```python
from build123d import *

# Parameters (mm, degrees)
SKETCH2_W                = 12.5
SKETCH2_H                = 12.5
SKETCH2_W_2              = 11.1
SKETCH2_H_2              = 11.1
BOSS_EXTRUDE1_DEPTH      = 105
SKETCH3_R                = 4
CUT_EXTRUDE1_DEPTH       = 105
SKETCH4_W                = 10
SKETCH4_H                = 2
BOSS_EXTRUDE2_DEPTH      = 25
FILLET1_R                = 5
SKETCH5_R                = 2
CUT_EXTRUDE2_DEPTH       = 40
BOSS_EXTRUDE3_START      = -82.5
SKETCH6_R                = 4
BOSS_EXTRUDE3_DEPTH      = 90.5
SKETCH8_W                = 12.5
SKETCH8_H                = 12.5
SKETCH8_W_2              = 11.1
SKETCH8_H_2              = 11.1
BOSS_EXTRUDE4_DEPTH      = 24
BOSS_EXTRUDE5_DEPTH      = 10
BOSS_EXTRUDE5_DEPTH_BACK = 51.049582
SKETCH9_W                = 12.5
SKETCH9_H                = 12.5
SKETCH9_W_2              = 10
SKETCH9_H_2              = 10
SKETCH11_R               = 4
BOSS_EXTRUDE6_DEPTH      = 11
SKETCH12_R               = 4
BOSS_EXTRUDE7_DEPTH      = 11


with BuildPart() as part:
    # Sketch2 → Boss-Extrude1 (new body)
    with BuildSketch(Plane.XY):
        Rectangle(SKETCH2_W, SKETCH2_H)
        Rectangle(SKETCH2_W_2, SKETCH2_H_2, mode=Mode.SUBTRACT)
    extrude(amount=BOSS_EXTRUDE1_DEPTH)

    # Sketch3 → Cut-Extrude1 (cut)
    with BuildSketch(Plane(origin=(0, 6.25, 0), x_dir=(1, 0, 0), z_dir=(0, 1, 0))):
        with Locations(Location((0, -95, 0), (0, 0, 180))):
            Circle(SKETCH3_R)
    extrude(amount=-CUT_EXTRUDE1_DEPTH, mode=Mode.SUBTRACT)

    # Sketch4 → Boss-Extrude2 (add, symmetric)
    with BuildSketch(Plane(origin=(0, 0, 0), x_dir=(0, 0, -1), z_dir=(1, 0, 0))):
        with Locations((-5, 0)):
            Rectangle(SKETCH4_W, SKETCH4_H)
    extrude(amount=BOSS_EXTRUDE2_DEPTH, both=True)

    # Fillet1
    fillet1_edges = [part.edges().sort_by_distance(p)[0] for p in [
        (-25, 0, 10),
        (-25, 0, 0),
        (25, 0, 10),
        (25, 0, 0),
    ]]
    fillet(fillet1_edges, radius=FILLET1_R - 0.0001)  # a hair under: the kernel refuses the full size

    # Sketch5 → Cut-Extrude2 (cut)
    with BuildSketch(Plane(origin=(0, 1, 0), x_dir=(1, 0, 0), z_dir=(0, 1, 0))):
        with Locations(Location((20, -5, 0), (0, 0, 270))):
            Circle(SKETCH5_R)
    cut_extrude2 = extrude(amount=-CUT_EXTRUDE2_DEPTH, mode=Mode.SUBTRACT)

    # Mirror1: Cut-Extrude2 across plane
    add(cut_extrude2.mirror(Plane(origin=(0, 0, 0), x_dir=(0, 0, 1), z_dir=(1, 0, 0))), mode=Mode.SUBTRACT)


with BuildPart() as body_2:
    # Mirror3: mirrored copy
    add(part.part.mirror(Plane(origin=(0, -75, 0), x_dir=(0, 0, 1), z_dir=(0, -1, 0))))



with BuildPart() as part_1:
    add(part.part)

    # Sketch6 → Boss-Extrude3 (add)
    with BuildSketch(Plane(origin=(0, 6.25, 0), x_dir=(1, 0, 0), z_dir=(0, 1, 0)).offset(BOSS_EXTRUDE3_START)):
        with Locations(Location((0, -43, 0), (0, 0, 180))):
            Circle(SKETCH6_R)
    boss_extrude3 = extrude(amount=BOSS_EXTRUDE3_DEPTH)

    # Mirror4: Boss-Extrude3 across plane
    add(boss_extrude3.mirror(Plane(origin=(0, -75, 0), x_dir=(0, 0, 1), z_dir=(0, -1, 0))))

    # Sketch8 → Boss-Extrude4 (add)
    with BuildSketch(Plane(origin=(0, 6.25, 0), x_dir=(1, 0, 0), z_dir=(0, 1, 0))):
        with Locations((0, -60.200417772)):
            Rectangle(SKETCH8_W, SKETCH8_H)
        with Locations((0, -60.200417772)):
            Rectangle(SKETCH8_W_2, SKETCH8_H_2, mode=Mode.SUBTRACT)
    extrude(amount=BOSS_EXTRUDE4_DEPTH)

    # Sketch9 → Boss-Extrude5 (add, two sides: drawn at the far end of the back side and taken through both)
    with BuildSketch(Plane(origin=(0, 0, 53.950417772), x_dir=(-1, 0, 0), z_dir=(0, 0, -1)).offset(-BOSS_EXTRUDE5_DEPTH_BACK)):
        with Locations((0, 36.5)):
            Rectangle(SKETCH9_W, SKETCH9_H)
        with Locations((0, 36.5)):
            Rectangle(SKETCH9_W_2, SKETCH9_H_2, mode=Mode.SUBTRACT)
    extrude(amount=BOSS_EXTRUDE5_DEPTH + BOSS_EXTRUDE5_DEPTH_BACK)

    # Sketch11 → Boss-Extrude6 (add, symmetric)
    with BuildSketch(Plane(origin=(0, 0, 0), x_dir=(1, 0, 0), z_dir=(0, 1, 0))):
        with Locations(Location((0, -95, 0), (0, 0, 180))):
            Circle(SKETCH11_R)
    extrude(amount=BOSS_EXTRUDE6_DEPTH, both=True)


with BuildPart() as body_2_1:
    add(body_2.part)

    add(part_1.part)  # Boss-Extrude7 merges part
    # Sketch12 → Boss-Extrude7 (add, symmetric)
    with BuildSketch(Plane(origin=(0, -150, 0), x_dir=(-1, 0, 0), z_dir=(0, -1, 0))):
        with Locations((0, -95)):
            Circle(SKETCH12_R)
    extrude(amount=BOSS_EXTRUDE7_DEPTH, both=True)


solid = body_2_1.part
```
Geometry: final body of the model. Coordinates: model frame, mm. A direction names the side the tool comes from. Coordinates: 2 decimals unless noted, no trailing zeros. Loops run counter-clockwise (first coordinate to the right, second up) from the corner with the lowest first, then second, coordinate; pieces in that order, holes last. Notation, with made-up numbers: (21.5, 4.25) -> (72.5, 4.25) arc R18 cw to (72.5, 9.25) -> close; hole circle Ø3 at (-28, 34.25). An arc over 180 degrees is marked (long way). Use a Markdown table: item, result. Add a question column.
(1) Section query A-A, the plane z = 51. Return loops of the section in (x, y), plus the area to 3 significant figures.
(2) Section query B-B, the plane x = -11. Return loops of the section in (y, z), plus the area to 3 significant figures.
(3) Line query: line 1 along Y through (x, z) = (-4.5, 46); line 2 along X through (y, z) = (-149.4, 5); line 3 along Y through (x, z) = (5.5, 16). Output: solid intervals per line, ascending.
(4) Section query D-D, the plane x = 0. State how many separate pieces and enclosed holes the cut face has, plus the area to 3 significant figures.
(5) Pin query (flat end, axial travel): pin 1 Ø9 at (x, y) = (1, 19) entering from +Z; pin 2 Ø10 at (x, y) = (0, 21) entering from -Z; pin 3 Ø10 at (x, y) = (0, -75.5) entering from -Z. Return the tip coordinate at first contact, or that it passes through.
(6) Access query for faces 4 (the cylindrical face through (-1.846, -8.592, 91.451)), 5 (the cylindrical face through (-1.846, -158.658, 98.549)), 6 (the flat face through (16, -149, 5)), 7 (the flat face through (-15, -1, 5)), 8 (the flat face through (0, 41.5, 75)). Directions: +Z, -Z, +X, -X, +Y, -Y. A direction counts if a zero-diameter tool reaches every point of the face in a straight line with its end or side. Return the directions, or none.
(7) Mould query, pull axis X, two halves, no side actions, for faces 1 (the cylindrical face through (-22, -150, 5)), 2 (the cylindrical face through (-24, 0, 2)), 3 (the flat face through (0, -11, 95)). Classes: pulls with the +X half, pulls with the -X half, needs draft (parallel to the pull), parting line crosses it, or undercut.
(8) Section query C-C, the plane y = -8.5. Return loops of the section in (x, z), plus the area to 3 significant figures.
Answer:
| question | item | result |
|---|---|---|
| 1 | outline | (-6.25, -156.25) -> (6.25, -156.25) -> (6.25, -143.75) -> (-6.25, -143.75) -> close; (-6.25, -6.25) -> (6.25, -6.25) -> (6.25, 6.25) -> (-6.25, 6.25) -> close; (-6.25, 30.25) -> (6.25, 30.25) -> (6.25, 42.75) -> (-6.25, 42.75) -> close; hole (-5.55, -155.55) -> (5.55, -155.55) -> (5.55, -144.45) -> (-5.55, -144.45) -> close; hole (-5.55, -5.55) -> (5.55, -5.55) -> (5.55, 5.55) -> (-5.55, 5.55) -> close; hole (-5, 31.5) -> (5, 31.5) -> (5, 41.5) -> (-5, 41.5) -> close |
| 1 | area | 122 mm^2 |
| 2 | outline | (-151, 0) -> (-149, 0) -> (-149, 10) -> (-151, 10) -> close; (-1, 0) -> (1, 0) -> (1, 10) -> (-1, 10) -> close |
| 2 | area | 40.0 mm^2 |
| 3 | line 1 | y = -156.25 to -155.55, -144.45 to -143.75, -6.25 to -5.55, 5.55 to 6.25, 30.25 to 31.5, 41.5 to 42.75 |
| 3 | line 2 | x = -25 to -22, -18 to 18, 22 to 25 |
| 3 | line 3 | y = -156.25 to -155.55, -144.45 to -143.75, -6.25 to -5.55, 5.55 to 6.25 |
| 4 | separate pieces | 4 |
| 4 | enclosed holes | 3 |
| 4 | area | 2,260 mm^2 |
| 5 | pin 1 | stops at z = 66.45 |
| 5 | pin 2 | stops at z = 53.95 |
| 5 | pin 3 | stops at z = 39 |
| 6 | face 4 | none |
| 6 | face 5 | -Y |
| 6 | face 6 | +Z, -Z, +X |
| 6 | face 7 | +Z, -Z, -X |
| 6 | face 8 | +Z, -Z |
| 7 | face 1 | undercut |
| 7 | face 2 | pulls with the -X half |
| 7 | face 3 | needs draft |
| 8 | outline | circle Ø8 at (0, 43); circle Ø8 at (0, 95) |
| 8 | area | 101 mm^2 |
